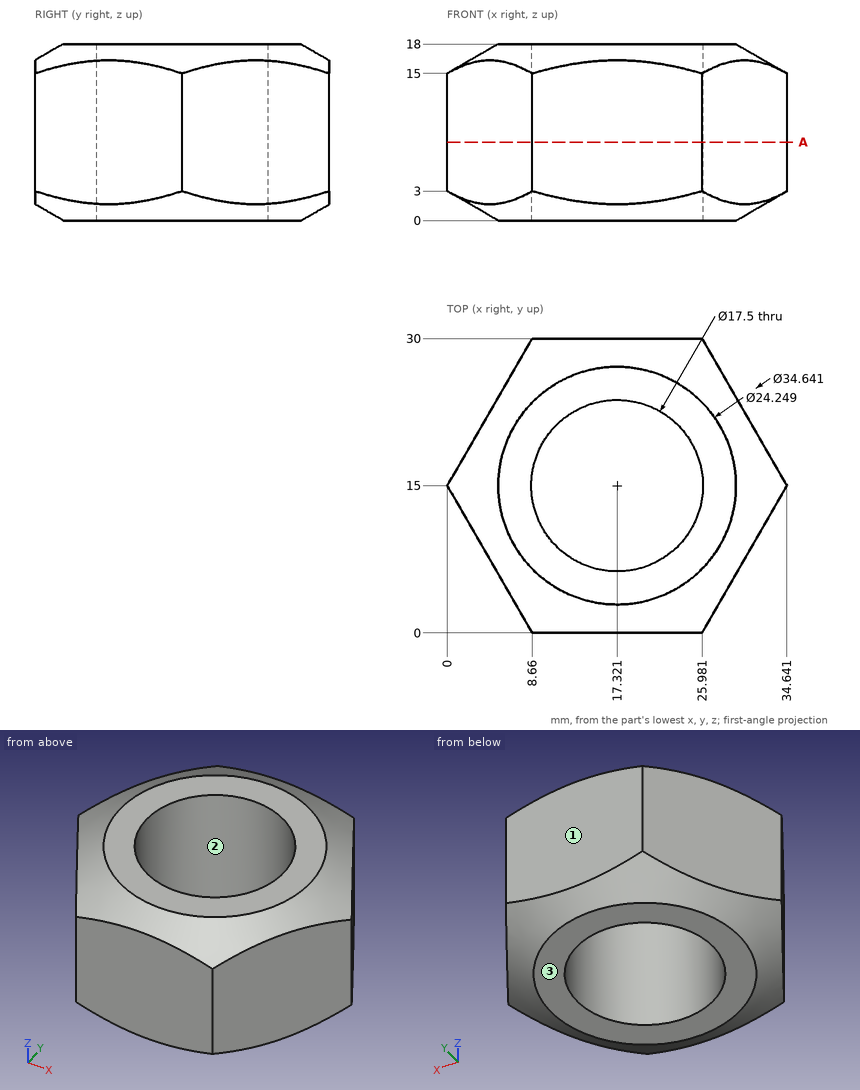
Check sheet for the drawn part. Datum: minimum x, y, z corner. Units: mm. Round coordinates to 2 decimals unless told otherwise and drop trailing zeros. Order: outer loops, then holes, each group sorted by start corner. A loop starts at its lowest first (then second) coordinate and runs counter-clockwise, first axis right, second up. Notation, with made-up numbers: (6, -32.5) -> (11, -32.5) arc R29 cw to (11, -9.5) -> close; hole circle Ø2 at (29.5, 56.25). An arc over 180 degrees is marked (long way). Put each result on its own line as item: value. Start each with the question number.
(1) Material ranges on line 1 along Y through (x, z) = (11, 3.5); line 2 along X through (y, z) = (6, 11.5) (1 decimal); line 3 along X through (y, z) = (14, 2) (1 decimal), recorded low to high.
(2) Draft check along Y on the marked faces 1, 2 and 3. Enter one of: +Y half, -Y half, draft (parallel to the pull), parting line (faces both ways), or undercut.
(3) Section check A-A (z = 8). Enter the section's corners in (x, y).
(4) Depth check by flat-ended pin: pin 1 Ø1.5 at (y, z) = (25.5, 15) entering from -X; pin 2 Ø6 at (y, z) = (7.5, 15.5) entering from -X; pin 3 Ø4 at (y, z) = (10.5, 5) entering from +X. Enter the tip coordinate at first touch or a pass-through.
Completed:
1. line 1: y = 0 to 8.95, 21.05 to 30
1. line 2: x = 5.2 to 29.4
1. line 3: x = 1.8 to 8.6, 26 to 32.9
2. face 1: +Y half
2. face 2: undercut
2. face 3: draft
3. outline: (0, 15) -> (8.66, 0) -> (25.98, 0) -> (34.64, 15) -> (25.98, 30) -> (8.66, 30) -> close; hole circle Ø17.5 at (17.32, 15)
4. pin 1: stops at x = 5.63
4. pin 2: stops at x = 2.6
4. pin 3: stops at x = 33.2
